```python
from build123d import *

# Parameters (mm, degrees)
EXTRUDE_1_DEPTH             = 90
SKETCH_2_W                  = 90
SKETCH_2_H                  = 42.75
EXTRUDE_2_DEPTH             = 8.2
SKETCH_3_W                  = 90
SKETCH_3_H                  = 52.45
EXTRUDE_3_DEPTH             = 8.2
SKETCH_4_W                  = 3.95
SKETCH_4_H                  = 2.25
CUT_EXTRUDE_1_DEPTH         = 235.487383722
SKETCH_5_W                  = 3.95
SKETCH_5_H                  = 29.5
CUT_EXTRUDE_2_DEPTH         = 235.487383722
SKETCH_6_W                  = 3.95
SKETCH_6_H                  = 6.2
CUT_EXTRUDE_3_DEPTH         = 235.487383722
SKETCH_7_W                  = 2.25
SKETCH_7_H                  = 3.95
CUT_EXTRUDE_4_DEPTH         = 235.487383722
SKETCH_8_W                  = 4.5
SKETCH_8_H                  = 3.95
CUT_EXTRUDE_5_DEPTH         = 235.487383722
SKETCH_9_W                  = 9
SKETCH_9_H                  = 3.95
CUT_EXTRUDE_6_DEPTH         = 235.487383722
SKETCH_10_W                 = 4.5
SKETCH_10_H                 = 3.95
CUT_EXTRUDE_7_DEPTH         = 235.487383722
SKETCH_11_W                 = 2.25
SKETCH_11_H                 = 3.95
CUT_EXTRUDE_8_DEPTH         = 235.487383722
SKETCH_12_W                 = 45.7
SKETCH_12_H                 = 44.2
CUT_EXTRUDE_9_DEPTH         = 86
HOLE_WIZARD_2_5_2_5_1_D     = 2.5
HOLE_WIZARD_4_5_4_5_1_D     = 4.5
HOLE_WIZARD_8_3_8_3_1_D     = 8.3
HOLE_WIZARD_8_3_8_3_1_DEPTH = 3.2
SKETCH_19_R                 = 1.67252853
SKETCH_19_R_2               = 1.459159852
SKETCH_19_R_3               = 1.459908976
SKETCH_19_R_4               = 1.592821911
SKETCH_19_R_5               = 1.532216665
SKETCH_19_R_6               = 1.596138091
EXTRUDE_4_DEPTH             = 90
CUT_EXTRUDE_START           = -90
SKETCH_20_R                 = 4.15
CUT_EXTRUDE_10_DEPTH        = 90
FILLET_1_R                  = 2
FILLET_2_R                  = 2
FILLET_3_R                  = 2
FILLET_4_R                  = 2
FILLET_5_R                  = 2
FILLET_6_R                  = 2
FILLET_7_R                  = 2
FILLET_8_R                  = 2
FILLET_9_R                  = 2
FILLET_10_R                 = 2
FILLET_11_R                 = 2
FILLET_12_R                 = 2
FILLET_13_R                 = 1.2


with BuildPart() as part:
    # Эскиз1 → Бобышка-Вытянуть1 (new body)
    with BuildSketch(Plane(origin=(90, 0, 0), x_dir=(0, 0, -1), z_dir=(1, 0, 0))):
        with BuildLine():
            Line((6.75, 160.906238208), (6.75, 204.25))
            Line((6.75, 204.25), (-38.093761792, 204.25))
            ThreePointArc((-38.093761792, 204.25), (-41.825, 203), (-38.093761792, 201.75))
            Line((-38.093761792, 201.75), (-37.5, 201.75))
            Line((-37.5, 201.75), (-37.5, 168.25))
            Line((-37.5, 168.25), (-38.093761792, 168.25))
            ThreePointArc((-38.093761792, 168.25), (-41.825, 167), (-38.093761792, 165.75))
            Line((-38.093761792, 165.75), (-37.5, 165.75))
            Line((-37.5, 165.75), (-37.5, 161.5))
            Line((-37.5, 161.5), (-33.25, 161.5))
            Line((-33.25, 161.5), (-33.25, 160.906238208))
            ThreePointArc((-33.25, 160.906238208), (-32, 157.175), (-30.75, 160.906238208))
            Line((-30.75, 160.906238208), (-30.75, 161.5))
            Line((-30.75, 161.5), (-22.25, 161.5))
            Line((-22.25, 161.5), (-22.25, 160.906238208))
            ThreePointArc((-22.25, 160.906238208), (-21, 157.175), (-19.75, 160.906238208))
            Line((-19.75, 160.906238208), (-19.75, 161.5))
            Line((-19.75, 161.5), (-6.75, 161.5))
            Line((-6.75, 161.5), (-6.75, 160.906238208))
            ThreePointArc((-6.75, 160.906238208), (-5.5, 157.175), (-4.25, 160.906238208))
            Line((-4.25, 160.906238208), (-4.25, 161.5))
            Line((-4.25, 161.5), (4.25, 161.5))
            Line((4.25, 161.5), (4.25, 160.906238208))
            ThreePointArc((4.25, 160.906238208), (5.5, 157.175), (6.75, 160.906238208))
        make_face()
    extrude(amount=-EXTRUDE_1_DEPTH)

    # Эскиз2 → Бобышка-Вытянуть2 (add)
    with BuildSketch(Plane(origin=(0, 0, -6.75), x_dir=(-1, 0, 0), z_dir=(0, 0, -1))):
        with Locations((-45, 182.875)):
            Rectangle(SKETCH_2_W, SKETCH_2_H)
    extrude(amount=EXTRUDE_2_DEPTH)

    # Эскиз3 → Бобышка-Вытянуть3 (add)
    with BuildSketch(Plane(origin=(0, 204.25, 0), x_dir=(-1, 0, 0), z_dir=(0, 1, 0))):
        with Locations((-45, 11.275)):
            Rectangle(SKETCH_3_W, SKETCH_3_H)
    extrude(amount=EXTRUDE_3_DEPTH)

    # Эскиз4 → Вырез-Вытянуть1 (cut, through all)
    with BuildSketch(Plane.ZY):
        with Locations((-12.975, 162.625)):
            Rectangle(SKETCH_4_W, SKETCH_4_H)
    extrude(amount=-CUT_EXTRUDE_1_DEPTH, mode=Mode.SUBTRACT)

    # Эскиз5 → Вырез-Вытянуть2 (cut, through all)
    with BuildSketch(Plane.ZY):
        with Locations((-12.975, 185)):
            Rectangle(SKETCH_5_W, SKETCH_5_H)
    extrude(amount=-CUT_EXTRUDE_2_DEPTH, mode=Mode.SUBTRACT)

    # Эскиз6 → Вырез-Вытянуть3 (cut, through all)
    with BuildSketch(Plane.ZY):
        with Locations((-12.975, 209.35)):
            Rectangle(SKETCH_6_W, SKETCH_6_H)
    extrude(amount=-CUT_EXTRUDE_3_DEPTH, mode=Mode.SUBTRACT)

    # Эскиз7 → Вырез-Вытянуть4 (cut, through all)
    with BuildSketch(Plane.ZY):
        with Locations((-9.875, 210.475)):
            Rectangle(SKETCH_7_W, SKETCH_7_H)
    extrude(amount=-CUT_EXTRUDE_4_DEPTH, mode=Mode.SUBTRACT)

    # Эскиз8 → Вырез-Вытянуть5 (cut, through all)
    with BuildSketch(Plane.ZY):
        with Locations((0, 210.475)):
            Rectangle(SKETCH_8_W, SKETCH_8_H)
    extrude(amount=-CUT_EXTRUDE_5_DEPTH, mode=Mode.SUBTRACT)

    # Эскиз9 → Вырез-Вытянуть6 (cut, through all)
    with BuildSketch(Plane.ZY):
        with Locations((13.25, 210.475)):
            Rectangle(SKETCH_9_W, SKETCH_9_H)
    extrude(amount=-CUT_EXTRUDE_6_DEPTH, mode=Mode.SUBTRACT)

    # Эскиз10 → Вырез-Вытянуть7 (cut, through all)
    with BuildSketch(Plane.ZY):
        with Locations((26.5, 210.475)):
            Rectangle(SKETCH_10_W, SKETCH_10_H)
    extrude(amount=-CUT_EXTRUDE_7_DEPTH, mode=Mode.SUBTRACT)

    # Эскиз11 → Вырез-Вытянуть8 (cut, through all)
    with BuildSketch(Plane.ZY):
        with Locations((36.375, 210.475)):
            Rectangle(SKETCH_11_W, SKETCH_11_H)
    extrude(amount=-CUT_EXTRUDE_8_DEPTH, mode=Mode.SUBTRACT)

    # Эскиз12 → Вырез-Вытянуть9 (cut)
    with BuildSketch(Plane(origin=(90, 0, 0), x_dir=(0, 0, -1), z_dir=(1, 0, 0))):
        with Locations((-13.25, 185)):
            Rectangle(SKETCH_12_W, SKETCH_12_H)
    extrude(amount=-CUT_EXTRUDE_9_DEPTH, mode=Mode.SUBTRACT)

    # Диаметр отверстия Ø2.5 (2.5)1 (through all)
    with Locations(Plane(origin=(90, 0, 0), x_dir=(0, 0, -1), z_dir=(1, 0, 0))):
        with Locations((5.5, 159.25), (-21, 159.25), (-5.5, 159.25), (-32, 159.25), (-39.75, 167), (-39.75, 203)):
            Hole(HOLE_WIZARD_2_5_2_5_1_D / 2)

    # Диаметр отверстия Ø4.5 (4.5)1 (through all)
    with Locations(Plane.ZY):
        with Locations((-13.25, 167), (-13.25, 203), (-5.5, 210.75), (5.5, 210.75), (21, 210.75), (32, 210.75)):
            Hole(HOLE_WIZARD_4_5_4_5_1_D / 2)

    # Диаметр отверстия Ø8.3 (8.3)1
    with Locations(Plane.ZY):
        with Locations((13.25, 185)):
            Hole(HOLE_WIZARD_8_3_8_3_1_D / 2, depth=HOLE_WIZARD_8_3_8_3_1_DEPTH)

    # Эскиз19 → Бобышка-Вытянуть4 (add)
    with BuildSketch(Plane(origin=(90, 0, 0), x_dir=(0, 0, -1), z_dir=(1, 0, 0))):
        with Locations((-39.75, 203)):
            Circle(SKETCH_19_R)
        with Locations((-39.75, 167)):
            Circle(SKETCH_19_R_2)
        with Locations((-32, 159.25)):
            Circle(SKETCH_19_R_3)
        with Locations((-21, 159.25)):
            Circle(SKETCH_19_R_4)
        with Locations((-5.5, 159.25)):
            Circle(SKETCH_19_R_5)
        with Locations((5.5, 159.25)):
            Circle(SKETCH_19_R_6)
    extrude(amount=-EXTRUDE_4_DEPTH)

    # Эскиз20 → Вырез-Вытянуть10 (cut)
    with BuildSketch(Plane.ZY.offset(CUT_EXTRUDE_START)):
        with Locations((13.25, 185)):
            Circle(SKETCH_20_R)
    extrude(amount=CUT_EXTRUDE_10_DEPTH, mode=Mode.SUBTRACT)

    # Скругление1
    fillet_1_edges = [part.edges().sort_by_distance(p)[0] for p in [
        (45, 208.5, -8.75),
    ]]
    fillet(fillet_1_edges, radius=FILLET_1_R)

    # Скругление2
    fillet_2_edges = [part.edges().sort_by_distance(p)[0] for p in [
        (45, 163.75, -11),
    ]]
    fillet(fillet_2_edges, radius=FILLET_2_R)

    # Скругление3
    fillet_3_edges = [part.edges().sort_by_distance(p)[0] for p in [
        (45, 170.25, -11),
    ]]
    fillet(fillet_3_edges, radius=FILLET_3_R)

    # Скругление4
    fillet_4_edges = [part.edges().sort_by_distance(p)[0] for p in [
        (45, 199.75, -11),
    ]]
    fillet(fillet_4_edges, radius=FILLET_4_R)

    # Скругление5
    fillet_5_edges = [part.edges().sort_by_distance(p)[0] for p in [
        (45, 206.25, -11),
    ]]
    fillet(fillet_5_edges, radius=FILLET_5_R)

    # Скругление6
    fillet_6_edges = [part.edges().sort_by_distance(p)[0] for p in [
        (45, 208.5, -2.25),
    ]]
    fillet(fillet_6_edges, radius=FILLET_6_R)

    # Скругление7
    fillet_7_edges = [part.edges().sort_by_distance(p)[0] for p in [
        (45, 208.5, 2.25),
    ]]
    fillet(fillet_7_edges, radius=FILLET_7_R)

    # Скругление8
    fillet_8_edges = [part.edges().sort_by_distance(p)[0] for p in [
        (45, 208.5, 8.75),
    ]]
    fillet(fillet_8_edges, radius=FILLET_8_R)

    # Скругление9
    fillet_9_edges = [part.edges().sort_by_distance(p)[0] for p in [
        (45, 208.5, 17.75),
    ]]
    fillet(fillet_9_edges, radius=FILLET_9_R)

    # Скругление10
    fillet_10_edges = [part.edges().sort_by_distance(p)[0] for p in [
        (45, 208.5, 24.25),
    ]]
    fillet(fillet_10_edges, radius=FILLET_10_R)

    # Скругление11
    fillet_11_edges = [part.edges().sort_by_distance(p)[0] for p in [
        (45, 208.5, 28.75),
    ]]
    fillet(fillet_11_edges, radius=FILLET_11_R)

    # Скругление12
    fillet_12_edges = [part.edges().sort_by_distance(p)[0] for p in [
        (45, 208.5, 35.25),
    ]]
    fillet(fillet_12_edges, radius=FILLET_12_R)

    # Скругление13
    fillet_13_edges = [part.edges().sort_by_distance(p)[0] for p in [
        (4, 185, -9.6),
        (4, 162.9, 13.25),
        (4, 185, 36.1),
        (4, 207.1, 13.25),
    ]]
    fillet(fillet_13_edges, radius=FILLET_13_R)


solid = part.part
```
The listing builds one solid part. Answer for the finished solid, in the listing's coordinates (mm). A direction names the side the tool comes from. Round coordinates to 2 decimals unless told otherwise and drop trailing zeros. Loops run counter-clockwise (first coordinate to the right, second up) from the corner with the lowest first, then second, coordinate; pieces in that order, holes last.
1) For a pull along Z with two mould halves and no side action, classify faces 5 (the face through (45.63, 206.82, -11.6)), 6 (the face through (45.63, 208.5, 32.08)), 7 (the face through (44, 199.75, -14)) as released by +Z, released by -Z, zero draft, split by the parting line, or undercut.
Outcome:
face 5: released by -Z
face 6: undercut
face 7: zero draft
2) A cutting plane is placed at B-B on y = 159.25. Determine the outline of the cut face in (x, z) (3 decimals).
Outcome:
outline: (0, -7.575) - (90, -7.575) - (90, -3.425) - (0, -3.425) - close; (0, 3.425) - (90, 3.425) - (90, 7.575) - (0, 7.575) - close; (0, 18.925) - (90, 18.925) - (90, 23.075) - (0, 23.075) - close; (0, 29.925) - (90, 29.925) - (90, 34.075) - (0, 34.075) - close
3) For faces 1 (the face through (44, 163.75, -14)), 2 (the face through (48, 207.1, 14)), 3 (the face through (46, 161.5, 0)), 4 (the face through (44, 211, -2.25)), determine the directions among +Z, -Z, +X, -X, +Y, -Y from which every point of the face is accessible in a straight line to the end or side of a thin tool.
Outcome:
face 1: -Z, +X, -X, -Y
face 2: +X
face 3: +X, -X
face 4: +X, -X, +Y
4) Consider line 1 (Y direction, x = 47.5, z = -13.25); line 2 (Z direction, x = 3.8, y = 185); line 3 (Y direction, x = 7.5, z = 26.5). Determine where each line is inside the solid, lowest interval first.
Outcome:
line 1: y = 163.75 to 164.75, 169.25 to 170.25, 199.75 to 200.75, 205.25 to 206.25
line 2: z = -11 to 9.1, 17.4 to 37.5
line 3: y = 161.5 to 162.9, 207.1 to 208.5
5) A cutting plane is placed at C-C on z = 5.5. Determine the outline of the cut face in (x, y) (3 decimals), plus the area to 3 significant figures.
Outcome:
outline: (0, 157.175) - (90, 157.175) - (90, 162.9) - (5.2, 162.9) arc R1.2 cw to (4, 164.1) - (4, 205.9) arc R1.2 cw to (5.2, 207.1) - (90, 207.1) - (90, 208.5) - (0, 208.5) - close
area: 819 mm2
6) Given P1, Ø0.7, axis at x = 47, z = 38, coming from the -Y side; P2, Ø2, axis at x = 49.5, y = 164.5, coming from the +Z side; P3, Ø4, axis at x = 62.5, y = 195.5, coming from the -Z side; P4, Ø3.5, axis at y = 167, z = -13.25, coming from the +X side, each flat-ended and moving along its own axis, determine where each tip first touches the part or whether it passes through.
Outcome:
P1: stops at y = 165.47
P2: stops at z = 41.18
P3: stops at z = -11
P4: passes through
7) A cutting plane is placed at A-A on z = 39.75. Determine the outline of the cut face in (x, y) (3 decimals), plus the area to 3 significant figures.
Outcome:
outline: (0, 164.925) - (90, 164.925) - (90, 169.075) - (0, 169.075) - close; (0, 200.925) - (90, 200.925) - (90, 205.075) - (0, 205.075) - close
area: 747 mm2
8) A cutting plane is placed at D-D on z = 13.5. Determine the outline of the cut face in (x, y).
Outcome:
outline: (0, 161.5) - (90, 161.5) - (90, 162.9) - (5.2, 162.9) arc R1.2 cw to (4, 164.1) - (4, 180.86) - (0, 180.86) - close; (0, 189.14) - (4, 189.14) - (4, 205.9) arc R1.2 cw to (5.2, 207.1) - (90, 207.1) - (90, 208.5) - (0, 208.5) - close
